Here's the drawing with two shaded views (mm, measured from the low corner). I have some questions. A direction names the side the tool comes from. Round coordinates to 2 decimals unless told otherwise and drop trailing zeros. Write each loop counter-clockwise with the first axis right and the second up, starting at its lowest first coordinate (ties: lowest second). Pieces come first, ordered by that corner, then holes. Notation, with made-up numbers: M 42,-18 L 83,-18 A18 ccw 83,-4 Z; hole C 32.5,-25.5 d10. An arc over 180 degrees is marked long. Write item = value, one per line. Start each with the question number.
(1) I want a section at C-C (z = 8). List the corners of the cut face in (x, y) for me.
(2) On a 3-axis mill with a long thin cutter (end or side, diameter ignored), from which of +Z, -Z, +X, -X, +Y, -Y can I reach the whole of each face in a straight line? I mean the marked faces 1 and 2. Say none if no direction works.
(3) I need wall thicknesses on line 1 along X through (y, z) = (43, 21); line 2 along Z through (x, y) = (31, 43); line 3 along X through (y, z) = (18.5, 21). Which ranges of each line are inside material? Lowest first, please.
(4) I want a section at B-B (z = 37). List the corners of the cut face in (x, y) for me, and give its area (3 significant figures).
(5) Will these pins go through, and if not, where does the flat tip stop? pin 1 Ø6 at (y, z) = (44.5, 44) entering from +X; pin 2 Ø1 at (y, z) = (30.5, 53.5) entering from -X; pin 3 Ø12 at (x, y) = (39.5, 47) entering from +Z.
(6) I want a section at A-A (x = 26.5). List the corners of the cut face in (y, z) for me.
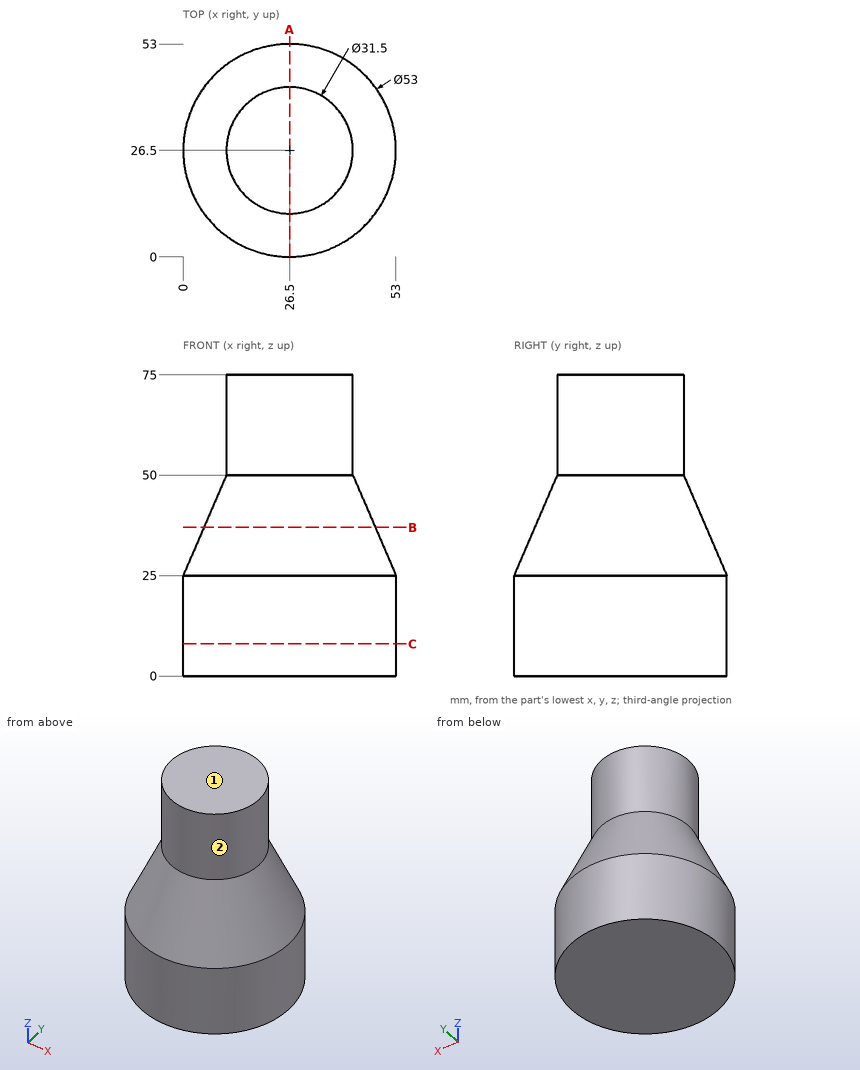
Returned:
q1.outline = C 26.5,26.5 d53
q2.face_1 = +Z, +X, -X, +Y, -Y
q2.face_2 = +Z
q3.line_1 = 5.76 to 47.24
q3.line_2 = 0 to 46.85
q3.line_3 = 1.24 to 51.76
q4.outline = C 26.5,26.5 d42.68
q4.area = 1,430 mm²
q5.pin_1 = 37.59
q5.pin_2 = 11.14
q5.pin_3 = 44.13
q6.outline = M 0,0 L 53,0 L 53,25 L 42.25,50 L 42.25,75 L 10.75,75 L 10.75,50 L 0,25 Z
